Read the model definition and answer for the solid it produces. Units are mm, in the model's axes. A direction names the side the tool comes from. Give positions to 0.01 mm unless a question says otherwise; leave off trailing zeros. Loops run counter-clockwise (first coordinate to the right, second up) from the corner with the lowest first, then second, coordinate; pieces in that order, holes last. Notation, with made-up numbers: (69, 51.25) -> (122, 51.25) arc R22 ccw to (122, 77.25) -> close; hole circle Ø6 at (68, 67.5). An arc over 180 degrees is marked (long way). Return JSON: item names as keys, results as strings. Group by question number.
from build123d import *

# Parameters (mm, degrees)
F0_R        = 7.5
F1_DEPTH    = 10
F3_DEPTH    = 7
F5_DEPTH    = 1
F6_T2_ANGLE = 299.893258673
F6_T4_ANGLE = 119.7759847122
F2_R        = 7.5
F2_R_2      = 6
F7_DEPTH    = 5
F8_DEPTH    = 5


# Not quite as in the source:
# - a fillet or chamfer that OpenCascade refuses, or shapes differently, is made with other operations: its cross-section is extruded or revolved along the edge and cut away or added


with BuildPart() as f1:
    # F0 (on Top) → F1 (new body)
    with BuildSketch(Plane.XY):
        Circle(F0_R)
    extrude(amount=F1_DEPTH)

    # F2 (on face) → F3 (cut)
    with BuildSketch(Plane.XY.offset(10)):
        with BuildLine():
            Line((-4.4899339722, 0.3008204206), (4.4899339722, 0.3008204206))
            ThreePointArc((4.4899339722, 0.3008204206), (0, 4.5), (-4.4899339722, 0.3008204206))
        make_face()
        with BuildLine():
            ThreePointArc((-4.4955897828, -0.1991795794), (0, -4.5), (4.4955897828, -0.1991795794))
            Line((4.4955897828, -0.1991795794), (-4.4955897828, -0.1991795794))
        make_face()
    extrude(amount=-F3_DEPTH, mode=Mode.SUBTRACT)

    # F4 (on face) → F5 (cut)
    with BuildSketch(Plane(origin=(0, 0, 0), x_dir=(1, 0, 0), z_dir=(0, 0, -1))):
        with BuildLine():
            Line((-1.1, -1), (-1.1, -7.4188947964))
            ThreePointArc((-1.1, -7.4188947964), (0, -7.5), (1.1, -7.4188947964))
            Line((1.1, -7.4188947964), (1.1, -1))
            Line((1.1, -1), (0, -1))
            Line((0, -1), (-1.1, -1))
        make_face()
    extrude(amount=-F5_DEPTH, mode=Mode.SUBTRACT)

    # F6: fillet of radius 2 on 1 edges, made by hand

    # F6_s1 → F6_t2 (revolve, cut)
    with BuildSketch(Plane(origin=(0, 0, 0), x_dir=(0, 0, 1), z_dir=(0.8669553942, -0.4983857387, 0))):
        with BuildLine():
            ThreePointArc((2, -7.5), (0.5857864376, -6.9142135624), (0, -5.5))
            Line((0, -5.5), (0, -7.5))
            Line((0, -7.5), (2, -7.5))
        make_face()
    revolve(axis=Axis((0, 0, 0), (0, 0, 1)), revolution_arc=F6_T2_ANGLE, mode=Mode.SUBTRACT)

    # F6_s3 → F6_t4 (revolve, cut)
    with BuildSketch(Plane.XZ):
        with BuildLine():
            ThreePointArc((7.5, 2), (6.9142135624, 0.5857864376), (5.5, 0))
            Line((5.5, 0), (7.5, 0))
            Line((7.5, 0), (7.5, 2))
        make_face()
    revolve(axis=Axis((0, 0, 0), (0, 0, 1)), revolution_arc=F6_T4_ANGLE, mode=Mode.SUBTRACT)

    # F2 (on face) → F7 (join)
    with BuildSketch(Plane.XY.offset(10)):
        Circle(F2_R)
        Circle(F2_R_2, mode=Mode.SUBTRACT)
    extrude(amount=F7_DEPTH)

    # F8 (add): a face of the model
    f8_faces = [f1.faces().sort_by_distance(p)[0] for p in [
        (-7.2878679656, 0, 15),
    ]]
    extrude(f8_faces, amount=F8_DEPTH)


solid = f1.part
1. Which of the six approach directions +Z, -Z, +X, -X, +Y, -Y give full straight-line access (tool end or side, diameter ignored) to faces 4 (the flat face through (0, 2, 3)), 5 (the flat face through (1.1, 4.1, 0.5)), 6 (the flat face through (0, 0, 0))?
2. Determine the mould class of faces 1 (the flat face through (0, -0.199, 7)), 2 (the flat face through (0, 1, 0.5)), 3 (the flat face through (2, 6, 20)) for opening direction Y: pulls with the +Y half, pulls with the -Y half, needs draft (parallel to the pull), parting line crosses it, or undercut.
3. Section B-B on z = 13.5 is taken. Determine the outline of the cut face in (x, y), then the cut area to 3 significant figures.
4. Flat-ended cylindrical pins translate along their axes: pin 1 Ø1.5 at (x, z) = (-2.5, 12.5) entering from +Y; pin 2 Ø3 at (x, z) = (-4.5, 2.5) entering from -Y; pin 3 Ø4 at (x, z) = (-3.5, 14) entering from -Y. Find the tip coordinate at first contact, or state that the pin passes through.
5. Straight lines are drawn through the part: line 1 (Y direction, x = 0, z = 15); line 2 (Y direction, x = -3, z = 6); line 3 (Y direction, x = 1, z = 4.5). For each, find the intervals that lie inside material, in ascending order. Write a range as from..to.
Completed:
{
 "1": {"face 4": "+Z", "face 5": "-Z, +Y", "face 6": "-Z, +X, -X, +Y, -Y"},
 "2": {"face 1": "undercut", "face 2": "pulls with the +Y half", "face 3": "needs draft"},
 "3": {"outline": "circle Ø15 at (0, 0); hole circle Ø12 at (0, 0)", "area": "63.6 mm²"},
 "4": {"pin 1": "stops at y = 7.29", "pin 2": "stops at y = -6.87", "pin 3": "stops at y = -7.35"},
 "5": {"line 1": "y = -7.5..-6, 6..7.5", "line 2": "y = -6.87..-3.35, -0.2..0.3, 3.35..6.87", "line 3": "y = -7.43..-4.39, -0.2..0.3, 4.39..7.43"}
}
